from build123d import *

# Parameters (mm, degrees)
SKETCH1_R                          = 19.3637
SKETCH1_R_2                        = 14.3637
MOTOR_FACE_AND_SCREW_EXTRUDE_DEPTH = 6.35
BOSS_EXTRUDE4_START                = 2
SKETCH7_R                          = 19.3637
SKETCH7_R_2                        = 15.6337
BOSS_EXTRUDE4_DEPTH                = 2
SKETCH3_R                          = 4.2
BOSS_EXTRUDE3_DEPTH                = 4
BOSS_EXTRUDE5_REACH                = 62.384
BOSS_EXTRUDE5_END_RADIUS           = 19.3637
SKETCH8_W                          = 8.35
SKETCH8_H                          = 38.7274
CHAMFER1_SIZE                      = 10
FILLET1_R                          = 5
SKETCH6_W                          = 7.14375
SKETCH6_H                          = 40.7637
F_1_0MM_DOWEL_HOLE1_AT_2_COUNT     = 2
F_1_0MM_DOWEL_HOLE1_AT_2_PITCH     = 60


with BuildPart() as part:
    # Sketch1 → Motor face and screw extrude (new body)
    with BuildSketch(Plane(origin=(0, 0, 0), x_dir=(0, 0, -1), z_dir=(1, 0, 0))):
        with Locations((0, -7)):
            Circle(SKETCH1_R)
        with Locations((0, -7)):
            Circle(SKETCH1_R_2, mode=Mode.SUBTRACT)
    extrude(amount=MOTOR_FACE_AND_SCREW_EXTRUDE_DEPTH)

    # Sketch7 → Boss-Extrude4 (add)
    with BuildSketch(Plane.ZY.offset(BOSS_EXTRUDE4_START)):
        with Locations((0, -7)):
            Circle(SKETCH7_R)
        with Locations((0, -7)):
            Circle(SKETCH7_R_2, mode=Mode.SUBTRACT)
    extrude(amount=-BOSS_EXTRUDE4_DEPTH)



with BuildPart() as body_2:
    # Sketch3 → Boss-Extrude3 (new body)
    with BuildSketch(Plane(origin=(0, -32.4, 0), x_dir=(1, 0, 0), z_dir=(0, 1, 0))):
        with BuildLine():
            Line((-12.7, -30), (-12.7, 30))
            ThreePointArc((-12.7, 30), (0, 42.7), (12.7, 30))
            Line((12.7, 30), (12.7, -30))
            ThreePointArc((12.7, -30), (0, -42.7), (-12.7, -30))
        make_face()
        with Locations(Location((0, 30, 0), (0, 0, 270))):
            Circle(SKETCH3_R, mode=Mode.SUBTRACT)
        with Locations(Location((0, -30, 0), (0, 0, 90))):
            Circle(SKETCH3_R, mode=Mode.SUBTRACT)
    extrude(amount=BOSS_EXTRUDE3_DEPTH)


with BuildPart() as part_1:
    add(part.part)

    add(body_2.part)  # Boss-Extrude5 merges body 2
    # Boss-Extrude5: up to this cylinder (the profile starts outside it)
    boss_extrude5_end = Plane(origin=(2.175, -7, 0), z_dir=(-1, 0, 0)) * Cylinder(BOSS_EXTRUDE5_END_RADIUS, 164.4954, mode=Mode.PRIVATE)
    # Sketch8 → Boss-Extrude5 (add, up to the surface)
    with BuildSketch(Plane(origin=(0, -28.4, 0), x_dir=(1, 0, 0), z_dir=(0, 1, 0)), mode=Mode.PRIVATE) as boss_extrude5_sk1:
        with Locations((2.175, 0)):
            Rectangle(SKETCH8_W, SKETCH8_H)
    boss_extrude5_tool1 = extrude(boss_extrude5_sk1.sketch, amount=BOSS_EXTRUDE5_REACH, mode=Mode.PRIVATE) - boss_extrude5_end
    add(boss_extrude5_tool1.solids().sort_by_distance((2.175, -28.4, 0))[0])

    # Chamfer1
    # the kernel refuses this chamfer: 10 mm, written as the material it adds along each edge
    with BuildSketch(Plane(origin=(-2, -28.4, -19.3637), x_dir=(-0.9996219169112968, -0.027495876610586317, 0), z_dir=(0, 0, 1))) as chamfer1_piece_1_section:
        Polygon((CHAMFER1_SIZE * 0.999621916911, -CHAMFER1_SIZE * 0.0274958766106), (-CHAMFER1_SIZE * 0.0274958766106, -CHAMFER1_SIZE * 0.999621916911), (0, 0), align=None)
    chamfer1_piece_1 = extrude(amount=38.7274, mode=Mode.PRIVATE)
    chamfer1_piece_1 = chamfer1_piece_1 - Plane(origin=(-3.620762983, -7, 0), x_dir=(0, 0, 1), z_dir=(-1, 0, 0)) * Cylinder(15.6337, 118, mode=Mode.PRIVATE)
    add(chamfer1_piece_1)

    # Fillet1
    fillet1_edges = [part_1.edges().sort_by_distance(p)[0] for p in [
        (-2.825, -28.4, -19.3637),
        (6.35, -28.4, 0),
        (-2.825, -28.4, 19.3637),
    ]]
    fillet(fillet1_edges, radius=FILLET1_R)

    # Sketch6 → Ø1.0mm Dowel Hole1 (revolve, cut)
    with BuildSketch(Plane(origin=(0, -28.4, 30), x_dir=(0, 0, -1), z_dir=(1, 0, 0))):
        with Locations((3.571875, 20.38185)):
            Rectangle(SKETCH6_W, SKETCH6_H)
    f_1_0mm_dowel_hole1 = revolve(axis=Axis((0, -34.75, 30), (0, 1, 0)), mode=Mode.SUBTRACT)

    # Ø1.0mm Dowel Hole1 at 2: Ø1.0mm Dowel Hole1 ×2
    with Locations(*[(0, 0, -i * F_1_0MM_DOWEL_HOLE1_AT_2_PITCH) for i in range(1, F_1_0MM_DOWEL_HOLE1_AT_2_COUNT)]):
        add(f_1_0mm_dowel_hole1, mode=Mode.SUBTRACT)


solid = part_1.part
Read the model definition and answer for the solid it produces. Units are mm, in the model's axes. A direction names the side the tool comes from. Coordinates: 2 decimals unless noted, no trailing zeros. Loops run counter-clockwise (first coordinate to the right, second up) from the corner with the lowest first, then second, coordinate; pieces in that order, holes last. Notation, with made-up numbers: (-7.75, -12) - (33.25, -12) arc R17 cw to (33.25, 0) - close; hole circle Ø4 at (15.5, 39.5). An arc over 180 degrees is marked (long way). Answer in a Markdown table with one row per item.
Q1. For faces 1 (the flat face through (0, -20, -7)), 2 (the flat face through (6.35, -22, 0)), 3 (the flat face through (-2, 9, 2)), 4 (the flat face through (1, -15, 19.364)), determine the directions among +Z, -Z, +X, -X, +Y, -Y from which every point of the face is accessible in a straight line to the end or side of a thin tool.
Here are the results:
| item | result |
|---|---|
| face 1 | -X |
| face 2 | +Z, -Z, +X, +Y |
| face 3 | +Z, -Z, -X, +Y |
| face 4 | +Z, +X, -X, +Y |
Q2. Find section A-A on z = 0. Write down the section's boundary in (x, y), plus the area to 3 significant figures.
Here are the results:
| item | result |
|---|---|
| outline | (-12.7, -32.4) - (12.7, -32.4) - (12.7, -28.4) - (11.35, -28.4) arc R5 cw to (6.35, -23.4) - (6.35, -21.36) - (0, -21.36) - (0, -22.63) - (-6.23, -22.63) - (-12, -28.4) - (-12.7, -28.4) - close; (-2, 8.63) - (0, 8.63) - (0, 7.36) - (6.35, 7.36) - (6.35, 12.36) - (-2, 12.36) - close |
| area | 243 mm^2 |
Q3. Find section D-D on z = 32. Write down the section's boundary in (x, y).
Here are the results:
| item | result |
|---|---|
| outline | (-12.54, -32.4) - (-3.69, -32.4) - (-3.69, -28.4) - (-12.54, -28.4) - close; (3.69, -32.4) - (12.54, -32.4) - (12.54, -28.4) - (3.69, -28.4) - close |
Q4. Find section B-B on x = 2.25. Write down the section's boundary in (y, z).
Here are the results:
| item | result |
|---|---|
| outline | (-32.4, -42.5) - (-28.4, -42.5) - (-28.4, -33.55) - (-32.4, -33.55) - close; (-32.4, -26.45) - (-28.4, -26.45) - (-28.4, -23.22) - (-28.27, -23.22) arc R5 cw to (-23.4, -19.36) - (-7, -19.36) arc R19.36 ccw to (-7, 19.36) - (-23.4, 19.36) arc R5 cw to (-28.27, 23.22) - (-28.4, 23.22) - (-28.4, 26.45) - (-32.4, 26.45) - close; (-32.4, 33.55) - (-28.4, 33.55) - (-28.4, 42.5) - (-32.4, 42.5) - close; hole circle Ø28.73 at (-7, 0) |
Q5. The mould has two halves that part along X. Classify faces 5 (the flat face through (-12.7, -30, 0)), 6 (the cylindrical face through (-2.6, -30.4, -33.3)), 7 (the flat face through (1, -15, -19.364)): pulls with the +X half, pulls with the -X half, needs draft (parallel to the pull), parting line crosses it, or undercut.
Here are the results:
| item | result |
|---|---|
| face 5 | pulls with the -X half |
| face 6 | undercut |
| face 7 | needs draft |
Q6. Straight lines are drawn through the part: line 1 along X through (y, z) = (-30.4, 30); line 2 along Y through (x, z) = (3, 0); line 3 along Y through (x, z) = (0.25, -5). For each, find the intervals that lie inside material, in ascending order. Write a range as [from, to].
Here are the results:
| item | result |
|---|---|
| line 1 | x = [-12.7, -4.2], [4.2, 12.7] |
| line 2 | y = [-32.4, -21.36], [7.36, 12.36] |
| line 3 | y = [-32.4, -20.47], [6.47, 11.71] |
Q7. Find section C-C on y = 4.5. Write down the section's boundary in (x, z), plus the area to 3 significant figures.
Here are the results:
| item | result |
|---|---|
| outline | (-2, -15.58) - (6.35, -15.58) - (6.35, -8.61) - (0, -8.61) - (0, -10.59) - (-2, -10.59) - close; (-2, 10.59) - (0, 10.59) - (0, 8.61) - (6.35, 8.61) - (6.35, 15.58) - (-2, 15.58) - close |
| area | 109 mm^2 |
Q8. Given P1, Ø14.5, axis at x = -1.5, y = -13, coming from the -Z side; P2, Ø1, axis at x = -3.5, y = -24, coming from the -Z side; P3, Ø1.5, axis at x = -6.5, z = 13, coming from the +Y side, each flat-ended and moving along its own axis, determine where each tip first touches the part or whether it passes through.
Here are the results:
| item | result |
|---|---|
| P1 | stops at z = -19.36 |
| P2 | stops at z = -19.49 |
| P3 | stops at y = -22.15 |
